For this review, use the dimensioned drawing (mm, ordinates from the lowest corner) and the shaded views. Round coordinates to 2 decimals unless told otherwise and drop trailing zeros. Loops run counter-clockwise (first coordinate to the right, second up) from the corner with the lowest first, then second, coordinate; pieces in that order, holes last. Notation, with made-up numbers: (31, 42) -> (71, 42) arc R20 cw to (71, 80) -> close; hole circle Ø2 at (25, 34). An arc over 180 degrees is marked (long way). Answer as CSV lines item,"result". Start each with the question number.
(1) Take a section at B-B, the plane z = 3. Write out the cut boundary in (x, y).
(2) Take a section at A-A, the plane x = 14. Write out the cut boundary in (y, z), and give its area (3 significant figures).
(3) Take a section at C-C, the plane y = 1.25. Write out the cut boundary in (x, z).
(4) To check wall thickness, follow line 1 (Z direction, x = 117, y = 0.9); line 2 (X direction, y = 0.8, z = 77); line 3 (Z direction, x = 108.5, y = 1.6). State the ranges of each line that lie inside material, in increasing order. Write a range as from..to.
(5) For P1, Ø1, axis at y = 1, z = 44.5, coming from the +X side, flat-tipped, find the tip position at first contact; note if it passes through.
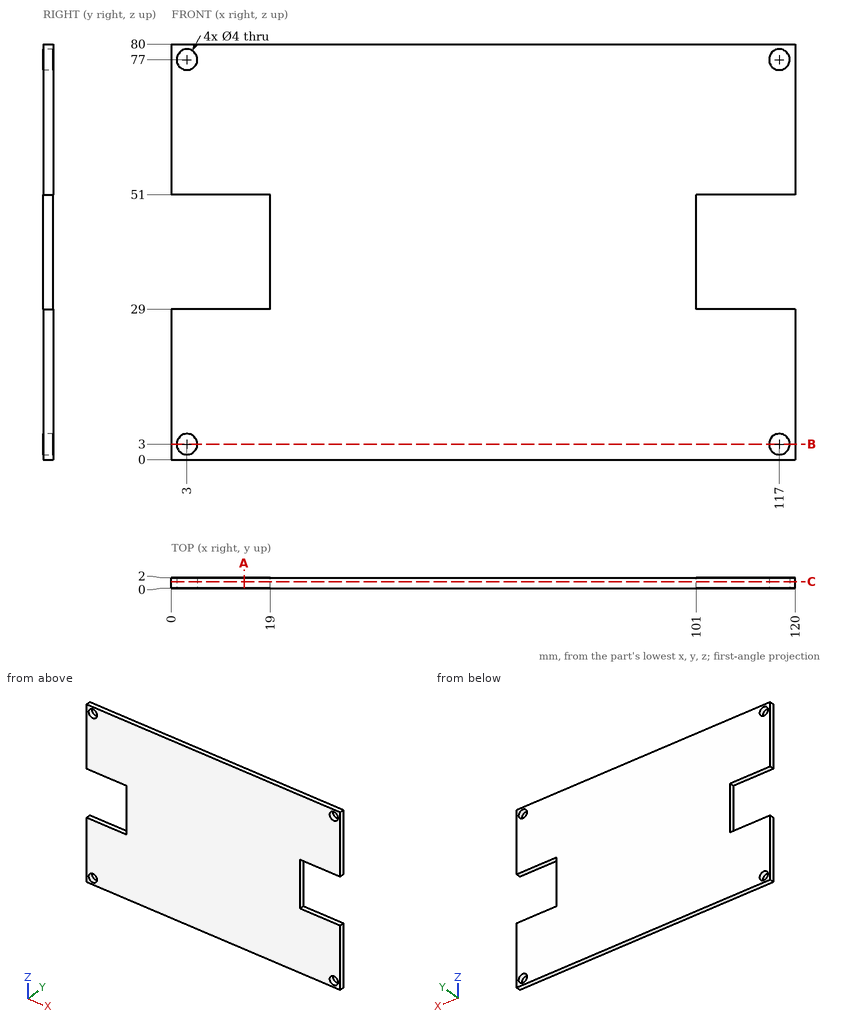
The answers:
1,outline,"(0, 0) -> (1, 0) -> (1, 2) -> (0, 2) -> close; (5, 0) -> (115, 0) -> (115, 2) -> (5, 2) -> close; (119, 0) -> (120, 0) -> (120, 2) -> (119, 2) -> close"
2,outline,"(0, 0) -> (2, 0) -> (2, 29) -> (0, 29) -> close; (0, 51) -> (2, 51) -> (2, 80) -> (0, 80) -> close"
2,area,"116 mm²"
3,outline,"(0, 0) -> (120, 0) -> (120, 29) -> (101, 29) -> (101, 51) -> (120, 51) -> (120, 80) -> (0, 80) -> (0, 51) -> (19, 51) -> (19, 29) -> (0, 29) -> close; hole circle Ø4 at (3, 3); hole circle Ø4 at (3, 77); hole circle Ø4 at (117, 3); hole circle Ø4 at (117, 77)"
4,line 1,"0..1, 5..29, 51..75, 79..80"
4,line 2,"0..1, 5..115, 119..120"
4,line 3,"0..29, 51..80"
5,P1,"x = 101"
